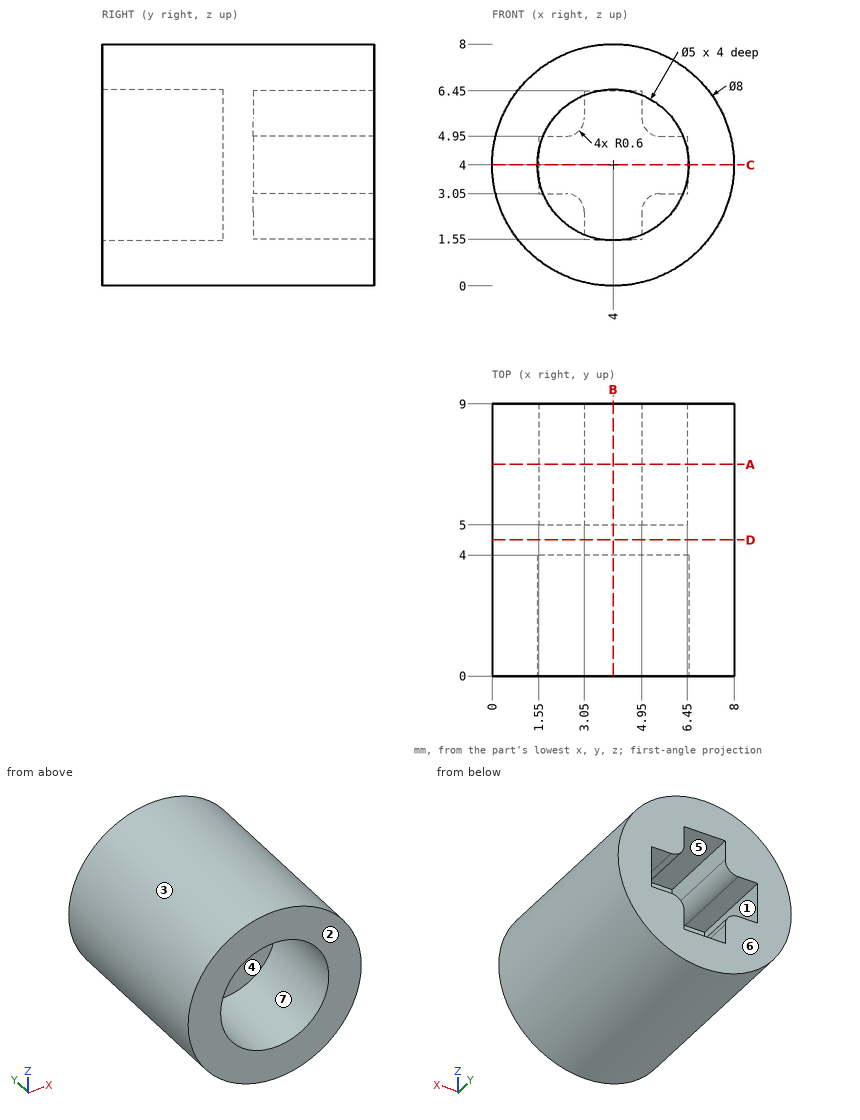
Verification items for this drawing (mm, ordinates from the low corner). A direction names the side the tool comes from. Give positions to 0.01 mm unless a question says otherwise; leave off trailing zeros. Write each loop counter-clockwise with the first axis right and the second up, starting at its lowest first coordinate (ties: lowest second). Pieces come first, ordered by that corner, then holes. Notation, with made-up numbers: (40, 2) - (92, 2) arc R20 cw to (92, 6) - close; hole circle Ø5 at (83.5, 48.5). An arc over 180 degrees is marked (long way). Answer as CSV lines item,"result". Start each with the question number.
1. Set-up check for the marked faces 5, 6 and 7: record each of +Z, -Z, +X, -X, +Y, -Y from which the full face is reachable in a straight line by a thin tool's end or side.
2. Sectioned sample at C-C (z = 4). Record the boundary of the cut face in (x, y), then the cut area to 3 significant figures.
3. Depth check by flat-ended pin: pin 1 (0.5 mm diameter, centred on x = 6, y = 7.5, fed in from -Z); pin 2 (0.5 mm diameter, centred on y = 7, z = 6, fed in from +X); pin 3 (0.5 mm diameter, centred on x = 2, y = 7, fed in from +Z). Enter the tip coordinate at first touch or a pass-through.
4. Sectioned sample at D-D (y = 4.5). Record the boundary of the cut face in (x, z).
5. Sectioned sample at B-B (x = 4). Record the boundary of the cut face in (y, z).
6. Thickness scan on line 1 (X direction, y = 1.5, z = 4); line 2 (Y direction, x = 2.25, z = 5); line 3 (Y direction, x = 5, z = 4.75). Record the ranges inside material, lowest first.
7. Sectioned sample at A-A (y = 7). Record the boundary of the cut face in (x, z).
8. Draft check along Z on the marked faces 1, 2, 3 and 4. Enter one of: pulls with the +Z half, pulls with the -Z half, needs draft (parallel to the pull), parting line crosses it, or undercut.
Derived:
1,face 5,"+Y"
1,face 6,"+Z, -Z, +X, -X, +Y"
1,face 7,"-Y"
2,outline,"(0, 0) - (1.5, 0) - (1.5, 4) - (6.5, 4) - (6.5, 0) - (8, 0) - (8, 9) - (6.45, 9) - (6.45, 5) - (1.55, 5) - (1.55, 9) - (0, 9) - close"
2,area,"32.4 mm²"
3,pin 1,"z = 0.4"
3,pin 2,"x = 7.6"
3,pin 3,"z = 7.6"
4,outline,"circle Ø8 at (4, 4)"
5,outline,"(0, 0) - (9, 0) - (9, 1.55) - (5, 1.55) - (5, 6.45) - (9, 6.45) - (9, 8) - (0, 8) - (0, 6.5) - (4, 6.5) - (4, 1.5) - (0, 1.5) - close"
6,line 1,"0 to 1.5, 6.5 to 8"
6,line 2,"4 to 9"
6,line 3,"4 to 5"
7,outline,"circle Ø8 at (4, 4); hole (1.55, 3.05) - (2.45, 3.05) arc R0.6 cw to (3.05, 2.45) - (3.05, 1.55) - (4.95, 1.55) - (4.95, 2.45) arc R0.6 cw to (5.55, 3.05) - (6.45, 3.05) - (6.45, 4.95) - (5.55, 4.95) arc R0.6 cw to (4.95, 5.55) - (4.95, 6.45) - (3.05, 6.45) - (3.05, 5.55) arc R0.6 cw to (2.45, 4.95) - (1.55, 4.95) - close"
8,face 1,"undercut"
8,face 2,"needs draft"
8,face 3,"parting line crosses it"
8,face 4,"undercut"
